```python
from build123d import *

# Parameters (mm, degrees)
BOSS_EXTRUDE1_DEPTH = 17
SKETCH4_OUTSIDE_W   = 84.788
SKETCH4_OUTSIDE_H   = 67.788
CUT_EXTRUDE1_DEPTH  = 15
FILLET4_R           = 2
FILLET5_R           = 2
SKETCH9_W           = 32
SKETCH9_H           = 2
CUT_EXTRUDE2_DEPTH  = 1
FILLET6_R           = 1
WRAP5_START         = 14
WRAP5_DEPTH         = 2


# Read off the part's stored shape, not the designer's step: Wrap5
with BuildPart() as part:
    # Sketch2 → Boss-Extrude1 (new body)
    with BuildSketch(Plane(origin=(0, 0, 0), x_dir=(1, 0, 0), z_dir=(0, 1, 0))):
        with BuildLine():
            Line((30.967741935, 8.062193214), (33, 0.25607376))
            Line((33, 0.25607376), (33, -17))
            Line((33, -17), (-33, -17))
            Line((-33, -17), (-33, 0.25607376))
            Line((-33, 0.25607376), (-30.967741935, 8.062193214))
            ThreePointArc((-30.967741935, 8.062193214), (0, 32), (30.967741935, 8.062193214))
        make_face()
    extrude(amount=BOSS_EXTRUDE1_DEPTH)

    # Sketch4 outside → Cut-Extrude1 (cut)
    # profile 1 of 2: a face of its own
    with BuildSketch(Plane(origin=(0, 17, 0), x_dir=(1, 0, 0), z_dir=(0, 1, 0))):
        with Locations((0, 7.5)):
            Rectangle(SKETCH4_OUTSIDE_W, SKETCH4_OUTSIDE_H)
        with BuildLine():
            Line((33, -17), (33, 0.25607376))
            Line((33, 0.25607376), (30.967741935, 8.062193214))
            ThreePointArc((30.967741935, 8.062193214), (0, 32), (-30.967741935, 8.062193214))
            Line((-30.967741935, 8.062193214), (-33, 0.25607376))
            Line((-33, 0.25607376), (-33, -17))
            Line((-33, -17), (33, -17))
        make_face(mode=Mode.SUBTRACT)
    # profile 2 of 2: a face of its own
    with BuildSketch(Plane(origin=(0, 17, 0), x_dir=(1, 0, 0), z_dir=(0, 1, 0))):
        with BuildLine():
            Line((-29.032258065, 7.558306138), (-31, 0))
            Line((-31, 0), (-31, -15))
            Line((-31, -15), (31, -15))
            Line((31, -15), (31, 0))
            Line((31, 0), (29.032258065, 7.558306138))
            ThreePointArc((29.032258065, 7.558306138), (0, 30), (-29.032258065, 7.558306138))
        make_face()
    extrude(amount=-CUT_EXTRUDE1_DEPTH, mode=Mode.SUBTRACT)

    # Fillet4
    fillet4_edges = [part.edges().sort_by_distance(p)[0] for p in [
        (33, 8.5, -0.25607376),
        (33, 8.5, 17),
        (-33, 8.5, 17),
        (-33, 8.5, -0.25607376),
        (31, 9.5, 0),
        (31, 9.5, 15),
        (-31, 9.5, 15),
        (-31, 9.5, 0),
    ]]
    fillet(fillet4_edges, radius=FILLET4_R)

    # Fillet5
    fillet5_edges = [part.edges().sort_by_distance(p)[0] for p in [
        (0, 2, -30),
        (-29.983870968, 2, -3.903059727),
        (0, 2, 15),
        (-31, 2, 6.62803688),
        (31, 2, 6.62803688),
        (29.983870968, 2, -3.903059727),
        (-30.983805401, 2, 0.002073506),
        (30.983805401, 2, 0.002073506),
        (30.414213562, 2, 14.414213562),
        (-30.414213562, 2, 14.414213562),
    ]]
    fillet(fillet5_edges, radius=FILLET5_R)

    # Sketch9 → Cut-Extrude2 (cut)
    with BuildSketch(Plane(origin=(0, 0, 15), x_dir=(-1, 0, 0), z_dir=(0, 0, -1))):
        with Locations((0, 15)):
            Rectangle(SKETCH9_W, SKETCH9_H)
    extrude(amount=-CUT_EXTRUDE2_DEPTH, mode=Mode.SUBTRACT)

    # Fillet6
    fillet6_edges = [part.edges().sort_by_distance(p)[0] for p in [
        (0, 16, 16),
    ]]
    fillet(fillet6_edges, radius=FILLET6_R - 0.0001)  # a hair under: the kernel refuses the full size
    fillet6_2_edges = [part.edges().sort_by_distance(p)[0] for p in [
        (-16, 14.50005, 16),
    ]]
    fillet(fillet6_2_edges, radius=FILLET6_R - 0.0001)  # a hair under: the kernel refuses the full size
    fillet6_3_edges = [part.edges().sort_by_distance(p)[0] for p in [
        (0.49995, 14, 16),
    ]]
    fillet(fillet6_3_edges, radius=FILLET6_R - 0.0001)  # a hair under: the kernel refuses the full size
    fillet6_4_edges = [part.edges().sort_by_distance(p)[0] for p in [
        (16, 15, 16),
    ]]
    fillet(fillet6_4_edges, radius=FILLET6_R - 0.0001)  # a hair under: the kernel refuses the full size

    # Wrap5 outline → Wrap5 (cut)
    with BuildSketch(Plane(origin=(0, 0, 0), x_dir=(1, 0, 0), z_dir=(0, 1, 0)).offset(WRAP5_START)):
        with BuildLine():
            Line((9.815840904, 28.348708389), (10.143035601, 29.293665336))
            ThreePointArc((10.143035601, 29.293665336), (0, 31), (-10.143035601, 29.293665336))
            Line((-10.143035601, 29.293665336), (-9.815840904, 28.348708389))
            ThreePointArc((-9.815840904, 28.348708389), (0, 30), (9.815840904, 28.348708389))
        make_face()
    extrude(amount=WRAP5_DEPTH, mode=Mode.SUBTRACT)


solid = part.part
```
Can you work these out from the model? Positions are in its coordinate system, mm. A direction names the side the tool comes from. Round coordinates to 2 decimals unless told otherwise and drop trailing zeros. Loops run counter-clockwise (first coordinate to the right, second up) from the corner with the lowest first, then second, coordinate; pieces in that order, holes last. Notation, with made-up numbers: M 26.5,68 L 71.5,68 A8 ccw 71.5,80 Z; hole C 57,58.5 d2. An arc over 180 degrees is marked long. Answer in a Markdown table with one row per item.
1. Please list where these lines run through material, in increasing order: line 1 (X direction, y = 10.75, z = 13.5); line 2 (X direction, y = 9, z = 11.5); line 3 (Y direction, x = 15.5, z = 10.5). Write a range as from..to.
Established:
| item | result |
|---|---|
| line 1 | -33..-30.94, 30.94..33 |
| line 2 | -33..-31, 31..33 |
| line 3 | 0..2 |
2. On a 3-axis mill with a long thin cutter (end or side, diameter ignored), from which of +Z, -Z, +X, -X, +Y, -Y can I reach the whole of each face in a straight line? I mean faces 1 (the face through (0, 0, -2)), 2 (the face through (0, 15, -31)), 3 (the face through (-30.43, 10.41, 14.4)). Say none if no direction works.
Established:
| item | result |
|---|---|
| face 1 | +Z, -Z, +X, -X, -Y |
| face 2 | none |
| face 3 | +Y |
3. If we section it at A-A, the plane y = 6.75: Please give me the cut outline in (x, z).
Established:
| item | result |
|---|---|
| outline | M -33,0 A2 ccw -32.94,-0.5 L -30.97,-8.06 A32 ccw 30.97,-8.06 L 32.94,-0.5 A2 ccw 33,0 L 33,15 A2 ccw 31,17 L -31,17 A2 ccw -33,15 Z; hole M -31,0.26 A2 ccw -30.94,-0.25 L -29.03,-7.56 A30 ccw 29.03,-7.56 L 30.94,-0.25 A2 ccw 31,0.26 L 31,13 A2 ccw 29,15 L -29,15 A2 ccw -31,13 Z |
4. If we section it at C-C, the plane y = 3: Please give me the cut outline in (x, z).
Established:
| item | result |
|---|---|
| outline | M -33,0 A2 ccw -32.94,-0.5 L -30.97,-8.06 A32 ccw 30.97,-8.06 L 32.94,-0.5 A2 ccw 33,0 L 33,15 A2 ccw 31,17 L -31,17 A2 ccw -33,15 Z; hole M -30.73,0.26 A1.73 ccw -30.68,-0.18 L -28.77,-7.49 A29.73 ccw 28.77,-7.49 L 30.68,-0.18 A1.73 ccw 30.73,0.26 L 30.73,13 A1.73 ccw 29,14.73 L -29,14.73 A1.73 ccw -30.73,13 Z |
5. Thinking about a two-plate mould opening in Z: for faces 4 (the face through (-29.97, 10.59, -3.95)), 5 (the face through (31.938, 8.381, -4.336)), 6 (the face through (32.43, 8.38, 16.4)), which applies, pulls with the +Z half, pulls with the -Z half, needs draft (parallel to the pull), parting line crosses it, or undercut?
Established:
| item | result |
|---|---|
| face 4 | undercut |
| face 5 | pulls with the -Z half |
| face 6 | pulls with the +Z half |
6. If we section it at B-B, the plane z = 3: Please give me the cut outline in (x, y).
Established:
| item | result |
|---|---|
| outline | M -33,0 L 33,0 L 33,17 L 31,17 L 31,4 A2 cw 29,2 L -29,2 A2 cw -31,4 L -31,17 L -33,17 Z |
7. I'm going to push flat-ended pins straight in: pin 1 Ø4 at (x, z) = (16, -3.5) entering from +Y; pin 2 Ø4 at (x, y) = (3.5, 8) entering from -Z; pin 3 Ø4 at (x, z) = (-16, -22.5) entering from +Y. Where does each tip first touch, or does it pass through?
Established:
| item | result |
|---|---|
| pin 1 | y = 2 |
| pin 2 | z = -31.96 |
| pin 3 | y = 2.81 |
